Build history of the part. All positions in model axes, mm. A direction names the side the tool comes from. Round coordinates to 2 decimals unless told otherwise and drop trailing zeros. Write each loop counter-clockwise with the first axis right and the second up, starting at its lowest first coordinate (ties: lowest second). Pieces come first, ordered by that corner, then holes. Notation, with made-up numbers: (83.5, 18.5) - (113.5, 18.5) arc R25 ccw to (113.5, 32.5) - close; hole circle Ø5 at (54, -7.5). An arc over 180 degrees is marked (long way). Write each question's results on one line, items separated by ' | '.
from build123d import *

# Parameters (mm, degrees)
F0_W      = 40
F0_H      = 38
F0_R      = 2.074
F0_W_2    = 10
F0_H_2    = 30
F1_DEPTH  = 10
F2_R      = 5
F3_R      = 2
F5_DEPTH  = 7.5
F6_R      = 5
F8_W      = 5
F8_H      = 45
F9_DEPTH  = 50
F7_R      = 2.074
F10_DEPTH = 25


with BuildPart() as f1:
    # F0 (on Top) → F1 (new body)
    with BuildSketch(Plane.XY):
        Rectangle(F0_W, F0_H)
        with Locations((-12.5, -11)):
            Circle(F0_R, mode=Mode.SUBTRACT)
        with Locations((12.5, -11)):
            Circle(F0_R, mode=Mode.SUBTRACT)
        with Locations((-12.5, 9)):
            Circle(F0_R, mode=Mode.SUBTRACT)
        Rectangle(F0_W_2, F0_H_2, mode=Mode.SUBTRACT)
        with Locations((12.5, 9)):
            Circle(F0_R, mode=Mode.SUBTRACT)
    extrude(amount=F1_DEPTH)

    # F2
    f2_edges = [f1.edges().sort_by_distance(p)[0] for p in [
        (-20, 19, 5),
        (20, 19, 5),
        (20, -19, 5),
        (-20, -19, 5),
    ]]
    fillet(f2_edges, radius=F2_R)

    # F3
    f3_edges = [f1.edges().sort_by_distance(p)[0] for p in [
        (-5, 15, 5),
        (5, 15, 5),
        (-5, -15, 5),
        (5, -15, 5),
    ]]
    fillet(f3_edges, radius=F3_R)

    # F4 (on Right) → F5 (join, symmetric)
    with BuildSketch(Plane.YZ):
        Polygon((42.293714, 96.933324), (4.293714, 96.933324), (-19, 10), (19, 10), align=None)
    extrude(amount=F5_DEPTH, both=True)

    # F6
    f6_edges = [f1.edges().sort_by_distance(p)[0] for p in [
        (-7.5, -7.353143, 53.466662),
        (7.5, -7.353143, 53.466662),
        (-7.5, 30.646857, 53.466662),
        (7.5, 30.646857, 53.466662),
    ]]
    fillet(f6_edges, radius=F6_R)

    # F8 (on Front) → F9 (cut, symmetric)
    with BuildSketch(Plane.XZ):
        with Locations((0, 22.5)):
            Rectangle(F8_W, F8_H)
    extrude(amount=F9_DEPTH, both=True, mode=Mode.SUBTRACT)

    # F7 (on Right) → F10 (cut, symmetric)
    with BuildSketch(Plane.YZ):
        with Locations((-2, 35)):
            Circle(F7_R)
        with Locations((6, 35)):
            Circle(F7_R)
    extrude(amount=F10_DEPTH, both=True, mode=Mode.SUBTRACT)


solid = f1.part
(1) Two-plate mould, pull along Y, no slides. Class faces 5 (the cylindrical face through (18, 18, 5)), 6 (the cylindrical face through (-12.95, -13.025, 4.93)), 7 (the flat face through (20, 0, 5)), 8 (the cylindrical face through (-4.43, 14.4, 5.07)): released by +Y, released by -Y, zero draft, split by the parting line, or undercut.
Worked answers:
face 5: released by +Y | face 6: undercut | face 7: zero draft | face 8: undercut
(2) Drill centre lines: probe 1 along Y at (x, z) = (-12.5, 5.5); probe 2 along X at (y, z) = (6, 40); probe 3 along Y at (x, z) = (5, 36). Where is each one in solid material? Low to high. Write a range as [from, to].
Worked answers:
probe 1: y = [-19, -13.07], [-8.93, 6.93], [11.07, 19] | probe 2: x = [-7.5, -2.5], [2.5, 7.5] | probe 3: y = [-11.34, -3.82], [-0.18, 4.18], [7.82, 25.27]
(3) Slice it at B-B, the plane y = -2. State how many separate pieces and enclosed holes the cut face has, and give its area (3 significant figures).
Worked answers:
separate pieces: 3 | enclosed holes: 0 | area: 994 mm2
(4) Slice it at A-A, the plane x = 12.5. Write the cut outline in (y, z).
Worked answers:
outline: (-19, 0) - (-13.07, 0) - (-13.07, 10) - (-19, 10) - close; (-8.93, 0) - (6.93, 0) - (6.93, 10) - (-8.93, 10) - close; (11.07, 0) - (19, 0) - (19, 10) - (11.07, 10) - close
(5) Tool access for faces 1 (the cylindrical face through (-4.4, -14.43, 5.07)), 2 (the flat face through (-7.5, 11, 54)), 3 (the flat face through (2.5, 4, 27)), 4 (the flat face through (9, 19, 5)): list every direction of +Z, -Z, +X, -X, +Y, -Y with a clear straight run to the whole face (end or side of a thin tool).
Worked answers:
face 1: -Z | face 2: +Z, -X, +Y, -Y | face 3: -Z, +Y, -Y | face 4: -Z, +X, -X, +Y
(6) Flat gauge pins, fed straight in: pin 1 Ø3.5 at (x, y) = (12.5, 9) entering from +Z; pin 2 Ø1.5 at (x, z) = (2, 46.5) entering from -Y; pin 3 Ø10 at (y, z) = (25.5, 60) entering from -X; pin 4 Ø10 at (y, z) = (-3, 78) entering from -X. Where does each tip first touch, or does it go through?
Worked answers:
pin 1: passes through | pin 2: stops at y = -9.42 | pin 3: stops at x = -7.5 | pin 4: stops at x = -7.02
